```python
from build123d import *

# Parameters (mm, degrees)
F3_DEPTH = 2.5
F6_SIZE  = 0.3


with BuildPart() as f1:
    # F0 (on Front) → F1 (revolve)
    with BuildSketch(Plane.XZ):
        Polygon((3.5, 4), (0, 4), (0, -4), (2, -4), (2, 0), (3.5, 0), align=None)
    revolve(axis=Axis((0, 0, 0), (0, 0, -1)))

    # F2 (on face) → F3 (cut)
    with BuildSketch(Plane.XY.offset(4)):
        Polygon((1.732051, 0), (0.866025, 1.5), (-0.866025, 1.5), (-1.732051, 0), (-0.866025, -1.5), (0.866025, -1.5), align=None)
    extrude(amount=-F3_DEPTH, mode=Mode.SUBTRACT)

    # F4 (on Front) → F5 (revolve, cut)
    with BuildSketch(Plane.XZ):
        with BuildLine():
            Line((0, 3.5), (0, 10))
            ThreePointArc((0, 10), (-3.25, 6.75), (0, 3.5))
        make_face()
    revolve(axis=Axis((0, 0, 3.375), (0, 0, -1)), mode=Mode.SUBTRACT)

    # F6
    f6_edges = [f1.edges().sort_by_distance(p)[0] for p in [
        (-3.5, 0, 4),
        (-3.5, 0, 0),
    ]]
    chamfer(f6_edges, length=F6_SIZE)


solid = f1.part
```
The listing builds one solid part. Answer for the finished solid, in the listing's coordinates (mm). A direction names the side the tool comes from. Give positions to 0.01 mm unless a question says otherwise; leave off trailing zeros. Write each loop counter-clockwise with the first axis right and the second up, starting at its lowest first coordinate (ties: lowest second). Pieces come first, ordered by that corner, then holes. Notation, with made-up numbers: M 79,75 L 137,75 A36 cw 137,114 Z; hole C 72.25,57 d9. An arc over 180 degrees is marked long. Write each question's results on one line, items separated by ' | '.
Q1. Consider L1, parallel to Z at x = -2.5, y = 0; L2, parallel to Z at x = 0.5, y = -0.75; L3, parallel to X at y = -1, z = -3.5. Determine where each line is inside the solid, lowest interval first. Write a range as from..to.
Output values:
L1: 0..4 | L2: -4..1.5 | L3: -1.73..1.73
Q2. Section C-C, the plane z = -2.5 is taken. Write down the section's boundary in (x, y).
Output values:
outline: C 0,0 d4
Q3. Section A-A, the plane z = 1.75 is taken. Write down the section's boundary in (x, y).
Output values:
outline: C 0,0 d7; hole M -1.73,0 L -0.87,-1.5 L 0.87,-1.5 L 1.73,0 L 0.87,1.5 L -0.87,1.5 Z
Q4. Section B-B, the plane x = 0 is taken. Write down the section's boundary in (y, z), then the cut area to 3 significant figures.
Output values:
outline: M -3.5,0.3 L -3.2,0 L -2,0 L -2,-4 L 2,-4 L 2,0 L 3.2,0 L 3.5,0.3 L 3.5,3.7 L 3.2,4 L 1.73,4 A3.25 cw 1.5,3.87 L 1.5,1.5 L -1.5,1.5 L -1.5,3.87 A3.25 cw -1.73,4 L -3.2,4 L -3.5,3.7 Z | area: 36.3 mm2
Q5. A tool of negligible diameter and unlimited length cuts with its end or side. For faces 1 (the cylindrical face through (0, 2, -2)), 2 (the flat face through (1.305, 0.74, 2.768)), 3 (the flat face through (1.4, 1.4, 4)), from which of +Z, -Z, +X, -X, +Y, -Y can it reach the whole face along a straight path? Write none if from no direction.
Output values:
face 1: -Z | face 2: +Z | face 3: +Z, +X, -X, +Y, -Y
Q6. Flat-ended cylindrical pins translate along their axes: P1, Ø2.5, axis at x = -0.5, y = 0.5, coming from the +Z side; P2, Ø1.5, axis at y = 1, z = 0, coming from the -X side; P3, Ø4, axis at x = -0.5, z = -3, coming from the -Y side; P4, Ø1.5, axis at y = -1.5, z = 3, coming from the -X side. Find the tip coordinate at first contact, or state that the pin passes through.
Output values:
P1: z = 4 | P2: x = -3.49 | P3: y = -2 | P4: x = -3.42
Q7. For a pull along X with two mould halves and no side action, classify faces 4 (the flat face through (0, -1.5, 3)), 5 (the cylindrical face through (3.233, 1.341, 2.024)), 6 (the flat face through (-2, 1, 0)) as released by +X, released by -X, zero draft, split by the parting line, or undercut.
Output values:
face 4: undercut | face 5: split by the parting line | face 6: zero draft
